Could you check a few things on this model? Use its own coordinates, in mm. Face numbers are marked on the shaded views. A direction names the side the tool comes from. Coordinates: 2 decimals unless noted, no trailing zeros. Loops run counter-clockwise (first coordinate to the right, second up) from the corner with the lowest first, then second, coordinate; pieces in that order, holes last. Notation, with made-up numbers: (35, 73) - (51, 73) arc R20 ccw to (51, 95) - close; hole circle Ø6 at (37, 9). An arc over 180 degrees is marked (long way). Put each result on its own line as item: value. Start each with the question number.
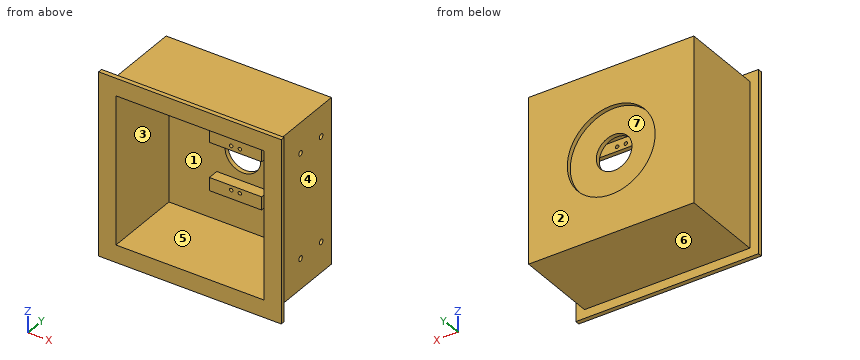
```python
from build123d import *

# Parameters (mm, degrees)
SKETCH1_W           = 210
SKETCH1_H           = 210
BOSS_EXTRUDE1_DEPTH = 5
SKETCH2_W           = 190
SKETCH2_H           = 190
BOSS_EXTRUDE2_DEPTH = 95
SKETCH3_W           = 170
SKETCH3_H           = 170
CUT_EXTRUDE1_DEPTH  = 90
SKETCH4_R           = 50.5
CUT_EXTRUDE2_DEPTH  = 5
SKETCH5_R           = 20.5
CUT_EXTRUDE3_DEPTH  = 5
SKETCH6_W           = 60
SKETCH6_H           = 15
BOSS_EXTRUDE3_DEPTH = 12.5
SKETCH7_W           = 50
SKETCH7_H           = 7.5
CUT_EXTRUDE4_DEPTH  = 12.5
SKETCH8_R           = 2
CUT_EXTRUDE5_DEPTH  = 7.5
SKETCH9_R           = 3
CUT_EXTRUDE6_DEPTH  = 7.5


with BuildPart() as part:
    # Sketch1 → Boss-Extrude1 (new body)
    with BuildSketch(Plane(origin=(0, 0, 0), x_dir=(1, 0, 0), z_dir=(0, 1, 0))):
        with Locations((-105, 105)):
            Rectangle(SKETCH1_W, SKETCH1_H)
    extrude(amount=BOSS_EXTRUDE1_DEPTH)

    # Sketch2 → Boss-Extrude2 (add)
    with BuildSketch(Plane(origin=(0, 5, 0), x_dir=(1, 0, 0), z_dir=(0, 1, 0))):
        with Locations((-105, 105)):
            Rectangle(SKETCH2_W, SKETCH2_H)
    extrude(amount=BOSS_EXTRUDE2_DEPTH)

    # Sketch3 → Cut-Extrude1 (cut)
    with BuildSketch(Plane(origin=(0, 0, 0), x_dir=(-1, 0, 0), z_dir=(0, -1, 0))):
        with Locations((105, 105)):
            Rectangle(SKETCH3_W, SKETCH3_H)
    extrude(amount=-CUT_EXTRUDE1_DEPTH, mode=Mode.SUBTRACT)

    # Sketch4 → Cut-Extrude2 (cut)
    with BuildSketch(Plane(origin=(0, 100, 0), x_dir=(1, 0, 0), z_dir=(0, 1, 0))):
        with Locations(Location((-105, 105, 0), (0, 0, 270))):
            Circle(SKETCH4_R)
    extrude(amount=-CUT_EXTRUDE2_DEPTH, mode=Mode.SUBTRACT)

    # Sketch5 → Cut-Extrude3 (cut)
    with BuildSketch(Plane(origin=(0, 95, 0), x_dir=(1, 0, 0), z_dir=(0, 1, 0))):
        with Locations(Location((-105, 105, 0), (0, 0, 270))):
            Circle(SKETCH5_R)
    extrude(amount=-CUT_EXTRUDE3_DEPTH, mode=Mode.SUBTRACT)

    # Sketch6 → Boss-Extrude3 (add)
    with BuildSketch(Plane.XZ.offset(-90)):
        with Locations((-105, -87.5)):
            Rectangle(SKETCH6_W, SKETCH6_H)
        with Locations((-105, -142.5)):
            Rectangle(SKETCH6_W, SKETCH6_H)
    extrude(amount=BOSS_EXTRUDE3_DEPTH)

    # Sketch7 → Cut-Extrude4 (cut)
    with BuildSketch(Plane(origin=(0, 0, -95), x_dir=(-1, 0, 0), z_dir=(0, 0, -1))):
        with Locations((105, 86.25)):
            Rectangle(SKETCH7_W, SKETCH7_H)
    extrude(amount=-CUT_EXTRUDE4_DEPTH, mode=Mode.SUBTRACT)

    # Sketch8 → Cut-Extrude5 (cut)
    with BuildSketch(Plane.XZ.offset(-77.5)):
        with Locations(Location((-100, -89.8, 0), (0, 0, 270))):
            Circle(SKETCH8_R)
        with Locations(Location((-110, -89.8, 0), (0, 0, 270))):
            Circle(SKETCH8_R)
        with Locations(Location((-110, -140.2, 0), (0, 0, 270))):
            Circle(SKETCH8_R)
        with Locations(Location((-100, -140.2, 0), (0, 0, 270))):
            Circle(SKETCH8_R)
    extrude(amount=-CUT_EXTRUDE5_DEPTH, mode=Mode.SUBTRACT)

    # Sketch9 → Cut-Extrude6 (cut)
    with BuildSketch(Plane(origin=(-10, 0, 0), x_dir=(0, 0, -1), z_dir=(1, 0, 0))):
        with Locations((165, 47.5)):
            Circle(SKETCH9_R)
        with Locations((45, 47.5)):
            Circle(SKETCH9_R)
        with Locations((45, 82.5)):
            Circle(SKETCH9_R)
        with Locations((165, 82.5)):
            Circle(SKETCH9_R)
    extrude(amount=-CUT_EXTRUDE6_DEPTH, mode=Mode.SUBTRACT)


solid = part.part
```
(1) I want a section at C-C on x = -195. List the corners of the cut face in (y, z) for me.
(2) I need wall thicknesses on L1, parallel to X at y = 81, z = -140; L2, parallel to Y at x = -12.75, z = -165; L3, parallel to X at y = 61, z = -122. Which ranges of each line are inside material? Lowest first, please. Write a range as [from, to].
(3) For pin 1 Ø10 at (x, z) = (-83.5, -152.5) entering from -Y; pin 2 Ø6.5 at (x, z) = (-100, -89.8) entering from +Y; pin 3 Ø7 at (y, z) = (47.5, -165) entering from +X, each with a flat end and sliding along its axis, tell me the tip position at first contact or that it passes through.
(4) Which directions (+Z, -Z, +X, -X, +Y, -Y) give clear straight access to the entire face, cutting with the end or side of a thin tool? Please do the marked faces 5, 6 and 7.
(5) I want a section at A-A on y = 10. List the corners of the cut face in (x, z) for me, and give its area (3 significant figures).
(6) I want a section at D-D on z = -32. List the corners of the cut face in (x, y) for me, and give its area (3 significant figures).
(7) I want a section at B-B on z = -105. List the corners of the cut face in (x, y) for me.
(8) If we mould it in two halves opening along X, with no side actions, what happens to the marked faces 1, 2, 3 and 4? For each: pulls with the +X half, pulls with the -X half, needs draft (parallel to the pull), parting line crosses it, or undercut.
Answer sheet:
1. outline: (0, -210) - (5, -210) - (5, -200) - (100, -200) - (100, -10) - (5, -10) - (5, 0) - (0, 0) - close
2. L1: x = [-200, -190], [-135, -111.99], [-108.01, -101.99], [-98.01, -75], [-20, -10]
2. L2: y = [0, 44.5], [50.5, 79.5], [85.5, 100]
2. L3: x = [-200, -190], [-20, -10]
3. pin 1: stops at y = 77.5
3. pin 2: stops at y = 82.5
3. pin 3: stops at x = -10
4. face 5: -Y
4. face 6: -Z, +X, -X, +Y
4. face 7: +Y
5. outline: (-200, -200) - (-10, -200) - (-10, -10) - (-200, -10) - close; hole (-190, -190) - (-20, -190) - (-20, -20) - (-190, -20) - close
5. area: 7,200 mm^2
6. outline: (-210, 0) - (-190, 0) - (-190, 90) - (-20, 90) - (-20, 0) - (0, 0) - (0, 5) - (-10, 5) - (-10, 100) - (-200, 100) - (-200, 5) - (-210, 5) - close
6. area: 3,800 mm^2
7. outline: (-210, 0) - (-190, 0) - (-190, 90) - (-125.5, 90) - (-125.5, 95) - (-155.5, 95) - (-155.5, 100) - (-200, 100) - (-200, 5) - (-210, 5) - close; (-84.5, 90) - (-20, 90) - (-20, 0) - (0, 0) - (0, 5) - (-10, 5) - (-10, 100) - (-54.5, 100) - (-54.5, 95) - (-84.5, 95) - close
8. face 1: undercut
8. face 2: needs draft
8. face 3: undercut
8. face 4: pulls with the +X half
